Input: part model. Units: mm. Frame: model coordinates. Face numbers are marked on the shaded views. A direction names the side the tool comes from. Give positions to 0.01 mm unless a question says otherwise; leave off trailing zeros. Loops run counter-clockwise (first coordinate to the right, second up) from the corner with the lowest first, then second, coordinate; pieces in that order, holes last. Notation, with made-up numbers: M -18.75,53 L 12.25,53 A25 ccw 12.25,68 Z; hole C 85.25,7 d6. An arc over 180 degrees is marked long. Answer as a JSON object with one key per item and string values. Group by question number.
1) First-contact query: P1, Ø3, axis at y = 0.5, z = 5.5, coming from the -X side; P2, Ø2, axis at x = 1, z = -3.5, coming from the -Y side. Flat tips, straight axial feed; report the tip coordinate or a pass-through.
2) Access query for the marked faces 3 and 4. Directions: +Z, -Z, +X, -X, +Y, -Y. A direction counts if a zero-diameter tool reaches every point of the face in a straight line with its end or side. Return the directions, or none.
3) Section query B-B on z = 5. Return loops of the section in (x, y), plus the area to 3 significant figures.
4) Draft query along Y for the marked faces 1 and 2. Return one class per face: +Y half, -Y half, draft (parallel to the pull), parting line (faces both ways), or undercut.
5) Ray query, L1, parallel to Z at x = 2.5, y = 1.25; L2, parallel to Z at x = 0.75, y = -0.75 (3 decimals); L3, parallel to X at y = 0.25, z = -6. Return the intervals inside material, ascending.
from build123d import *

# Parameters (mm, degrees)
EXTRUDE1_START     = -5.35
SKETCH1_R          = 2
EXTRUDE1_DEPTH     = 12
EXTRUDE2_START     = -6.65
SKETCH6_R          = 3.5
EXTRUDE2_DEPTH     = 1.3
CUT_EXTRUDE1_DEPTH = 0.975
SKETCH8_R          = 1.443375673
CUT_EXTRUDE2_DEPTH = 0.975
CUT_EXTRUDE2_TAPER = 45
CHAMFER1_SIZE      = 0.1625
CHAMFER2_SIZE      = 0.525


with BuildPart() as part:
    # Sketch1 → Extrude1 (new body)
    with BuildSketch(Plane.XY.offset(EXTRUDE1_START)):
        Circle(SKETCH1_R)
    extrude(amount=EXTRUDE1_DEPTH)

    # Sketch6 → Extrude2 (add)
    with BuildSketch(Plane.XY.offset(EXTRUDE2_START)):
        Circle(SKETCH6_R)
    extrude(amount=EXTRUDE2_DEPTH)

    # Sketch7 → Cut-Extrude1 (cut)
    with BuildSketch(Plane.XY.offset(-6.65)):
        Polygon((0, 1.443375673), (-1.25, 0.721687836), (-1.25, -0.721687836), (0, -1.443375673), (1.25, -0.721687836), (1.25, 0.721687836), align=None)
    extrude(amount=CUT_EXTRUDE1_DEPTH, mode=Mode.SUBTRACT)

    # Sketch8 → Cut-Extrude2 (cut)
    with BuildSketch(Plane.XY.offset(-6.65)):
        Circle(SKETCH8_R)
    extrude(amount=CUT_EXTRUDE2_DEPTH, taper=CUT_EXTRUDE2_TAPER, mode=Mode.SUBTRACT)

    # Chamfer1
    chamfer1_edges = [part.edges().sort_by_distance(p)[0] for p in [
        (-3.5, 0, -5.35),
        (-3.5, 0, -6.65),
    ]]
    chamfer(chamfer1_edges, length=CHAMFER1_SIZE)

    # Chamfer2
    chamfer2_edges = [part.edges().sort_by_distance(p)[0] for p in [
        (-2, 0, 6.65),
    ]]
    chamfer(chamfer2_edges, length=CHAMFER2_SIZE)


solid = part.part
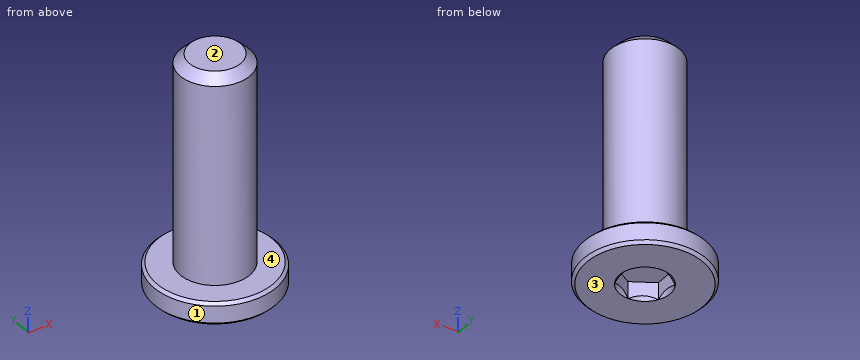
Output:
{
 "1": {"P1": "stops at x = -2", "P2": "stops at y = -2"},
 "2": {"face 3": "-Z, +X, -X, +Y, -Y", "face 4": "+Z"},
 "3": {"outline": "C 0,0 d4", "area": "12.6 mm^2"},
 "4": {"face 1": "parting line", "face 2": "draft"},
 "5": {"L1": "z = -6.65 to -5.35", "L2": "z = -5.675 to 6.65", "L3": "x = -3.49 to -1.25, 1.25 to 3.49"}
}
